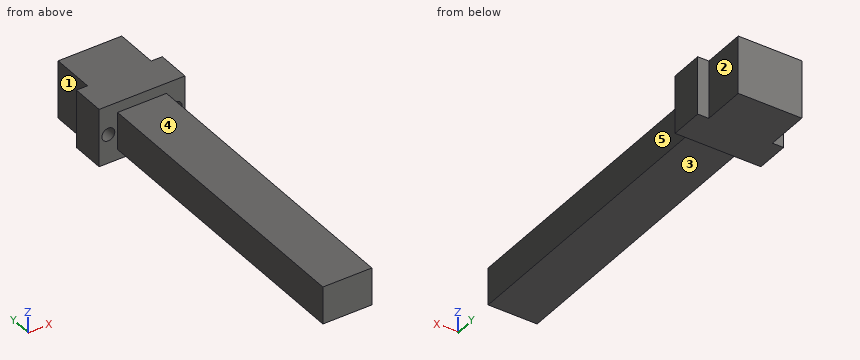
```python
from build123d import *

# Parameters (mm, degrees)
BOSS_EXTRUDE1_DEPTH = 21
SKETCH2_R           = 2.332714882
CUT_EXTRUDE1_DEPTH  = 11
CUT_EXTRUDE2_REACH  = 26.37
SKETCH3_W           = 3.734340962
SKETCH3_H           = 109.655613693


with BuildPart() as part:
    # Sketch1 → Boss-Extrude1 (new body)
    with BuildSketch(Plane.XY):
        Polygon((11.4999958, -2.86166347), (11.4999958, 12.851204158), (-11.4999958, 12.831547243), (-11.4999958, -2.86166347), (-15.520087877, -2.86166347), (-15.520087877, -14.967378119), (-11.520087877, -14.967378119), (-8.849574745, -14.967378119), (-8.849574745, -124.622991812), (8.849574745, -124.622991812), (8.849574745, -14.967378119), (11.520087877, -14.967378119), (15.520087877, -14.967378119), (15.520087877, -2.86166347), align=None)
    extrude(amount=BOSS_EXTRUDE1_DEPTH)

    # Sketch2 → Cut-Extrude1 (cut)
    with BuildSketch(Plane.XZ.offset(14.967378119)):
        with Locations((-12.184831311, 10.5)):
            Circle(SKETCH2_R)
        with Locations((12.184831311, 10.5)):
            Circle(SKETCH2_R)
    extrude(amount=-CUT_EXTRUDE1_DEPTH, mode=Mode.SUBTRACT)

    # Sketch3 → Cut-Extrude2 (cut, up to next)
    with BuildSketch(Plane.ZY.offset(8.849574745), mode=Mode.PRIVATE) as cut_extrude2_sk1:
        with Locations((19.132829519, -69.795184965)):
            Rectangle(SKETCH3_W, SKETCH3_H)
    cut_extrude2_tool1 = extrude(cut_extrude2_sk1.sketch, amount=-CUT_EXTRUDE2_REACH, mode=Mode.PRIVATE) & part.part
    add(cut_extrude2_tool1.solids().sort_by_distance((-8.849575, -69.795185, 19.13283))[0], mode=Mode.SUBTRACT)
    # Sketch3 → Cut-Extrude2 (cut, up to next)
    with BuildSketch(Plane.ZY.offset(8.849574745), mode=Mode.PRIVATE) as cut_extrude2_sk2:
        with Locations((1.867170481, -69.795184965)):
            Rectangle(SKETCH3_W, SKETCH3_H)
    cut_extrude2_tool2 = extrude(cut_extrude2_sk2.sketch, amount=-CUT_EXTRUDE2_REACH, mode=Mode.PRIVATE) & part.part
    add(cut_extrude2_tool2.solids().sort_by_distance((-8.849575, -69.795185, 1.86717))[0], mode=Mode.SUBTRACT)


solid = part.part
```
Build history of the part. All positions in model axes, mm. Face numbers are marked on the shaded views. A direction names the side the tool comes from. Give positions to 0.01 mm unless a question says otherwise; leave off trailing zeros. Order: outer loops, then holes, each group sorted by start corner. A loop starts at its lowest first (then second) coordinate and runs counter-clockwise, first axis right, second up. Notation, with made-up numbers: M 68.5,13.5 L 97.5,13.5 A20 cw 97.5,51.5 Z; hole C 62,13.25 d3. An arc over 180 degrees is marked long. Write item = value, one per line. Start each with the question number.
(1) Probe L1, parallel to Z at x = 1.5, y = -103; L2, parallel to Y at x = 6, z = 11.5; L3, parallel to Y at x = 0.5, z = 18. List the from-to ranges inside material, lowest first. Write a range as [from, to].
(2) Which spindle directions (+Z, -Z, +X, -X, +Y, -Y) get a long thin tool onto all of the face, cutting with end or side? Do the marked faces 1, 2, 3, 4 and 5. Say none if no direction does.
(3) Slice it at A-A on z = 18.5. Write the cut outline in (x, y), plus the area to 3 significant figures.
(4) Slice it at C-C on x = 13. Write the cut outline in (y, z).
(5) Slice it at D-D on y = -109. Write the cut outline in (x, z).
(6) Slice it at B-B on y = -9. Write the cut outline in (x, z).
(7) Pin check, flat tips, straight feed: pin 1 Ø8 at (y, z) = (7, 11) entering from -X; pin 2 Ø3 at (x, z) = (-12.18, 10.5) entering from -Y; pin 3 Ø1.2 at (x, z) = (14.5, 15.5) entering from +Y; pin 4 Ø5.5 at (x, z) = (12.18, 10.5) entering from +Y. Stop position of each tip, or through.
Responses:
q1.L1 = [3.73, 17.27]
q1.L2 = [-124.62, 12.85]
q1.L3 = [-14.97, 12.84]
q2.face_1 = +Z, -Z, -X, +Y
q2.face_2 = +Z, -Z, +X, +Y
q2.face_3 = -Z, +X, -X, -Y
q2.face_4 = +Z, +X, -X, -Y
q2.face_5 = +Z, -Z, +X, -Y
q3.outline = M -15.52,-14.97 L 15.52,-14.97 L 15.52,-2.86 L 11.5,-2.86 L 11.5,12.85 L -11.5,12.83 L -11.5,-2.86 L -15.52,-2.86 Z
q3.area = 737 mm2
q4.outline = M -14.97,0 L -2.86,0 L -2.86,21 L -14.97,21 L -14.97,12.69 L -3.97,12.69 L -3.97,8.31 L -14.97,8.31 Z
q5.outline = M -8.85,3.73 L 8.85,3.73 L 8.85,17.27 L -8.85,17.27 Z
q6.outline = M -15.52,0 L 15.52,0 L 15.52,21 L -15.52,21 Z; hole C -12.18,10.5 d4.67; hole C 12.18,10.5 d4.67
q7.pin_1 = -11.5
q7.pin_2 = -3.97
q7.pin_3 = -2.86
q7.pin_4 = 12.85
